from build123d import *

# Parameters (mm, degrees)
F0_R      = 31.75
F0_R_2    = 3.175
F1_DEPTH  = 12.7
F2_R      = 15.875
F2_R_2    = 9.525
F3_DEPTH  = 12.7
F3_FACE_R = 9.525
F4_DEPTH  = 25.4


with BuildPart() as f1:
    # F0 (on Top) → F1 (new body)
    with BuildSketch(Plane.XY):
        Circle(F0_R)
        with Locations((0, -25.4)):
            Circle(F0_R_2, mode=Mode.SUBTRACT)
        with Locations((-25.4, 0)):
            Circle(F0_R_2, mode=Mode.SUBTRACT)
        with Locations((25.4, 0)):
            Circle(F0_R_2, mode=Mode.SUBTRACT)
        with Locations((0, 25.4)):
            Circle(F0_R_2, mode=Mode.SUBTRACT)
    extrude(amount=F1_DEPTH)

    # F2 (on face) → F3 (join)
    with BuildSketch(Plane.XY.offset(12.7)):
        Circle(F2_R)
        Circle(F2_R_2, mode=Mode.SUBTRACT)
    extrude(amount=F3_DEPTH)

    # F3_face (on face) → F4 (cut)
    with BuildSketch(Plane.XY.offset(12.7)):
        Circle(F3_FACE_R)
    extrude(amount=-F4_DEPTH, mode=Mode.SUBTRACT)


solid = f1.part
Source: CAD feature listing. Evaluate the final solid. Frame: model axes, mm. A direction names the side the tool comes from. Round coordinates to 2 decimals unless told otherwise and drop trailing zeros. Write each loop counter-clockwise with the first axis right and the second up, starting at its lowest first coordinate (ties: lowest second). Pieces come first, ordered by that corner, then holes. Notation, with made-up numbers: (75.5, -0.5) - (82.5, -0.5) arc R20 ccw to (82.5, 19.5) - close; hole circle Ø3 at (8, 20). An arc over 180 degrees is marked (long way). Use CSV: the item, a comma, the result in double quotes. Start each with the question number.
(1) Material intervals for probe 1 along Y at (x, z) = (0, 9.75) (3 decimals); probe 2 along Y at (x, z) = (0, 22.75) (3 decimals); probe 3 along Z at (x, y) = (15, 22.5), sorted ascending. Write a range as [from, to].
(2) Cut plane D-D, the plane z = 8.75. Return loops of the section in (x, y) (3 decimals), and give its area (3 significant figures).
(3) Cut plane A-A, the plane x = 0. Return loops of the section in (y, z) (3 decimals).
(4) Mould query, pull axis X, two halves, no side actions, for faces 1 (the face through (7, 8, 0)), 2 (the face through (-0.41, -22.25, 6.26)), 3 (the face through (-3.441, -15.497, 18.961)). Classes: pulls with the +X half, pulls with the -X half, needs draft (parallel to the pull), parting line crosses it, or undercut.
(5) Set-up query: faces 4 (the face through (-6.883, -30.995, 6.261)), 5 (the face through (7, 15, 12.7)). Return all of +Z, -Z, +X, -X, +Y, -Y with unobstructed straight access to the full face (end or side cutting, diameter ignored); none if empty.
(6) Cut plane C-C, the plane x = -25.4. Return loops of the section in (y, z) (3 decimals).
(7) First-contact query: pin 1 Ø8.5 at (x, y) = (0, -25.4) entering from +Z; pin 2 Ø8 at (y, z) = (15.5, 6) entering from +X; pin 3 Ø12 at (y, z) = (15.5, 13) entering from -X. Flat tips, straight axial feed; report the tip coordinate or a pass-through.
Geometry says:
1,probe 1,"[-31.75, -28.575], [-22.225, -9.525], [9.525, 22.225], [28.575, 31.75]"
1,probe 2,"[-15.875, -9.525], [9.525, 15.875]"
1,probe 3,"[0, 12.7]"
2,outline,"circle Ø63.5 at (0, 0); hole circle Ø6.35 at (-25.4, 0); hole circle Ø19.05 at (0, 0); hole circle Ø6.35 at (0, -25.4); hole circle Ø6.35 at (0, 25.4); hole circle Ø6.35 at (25.4, 0)"
2,area,"2,760 mm²"
3,outline,"(-31.75, 0) - (-28.575, 0) - (-28.575, 12.7) - (-31.75, 12.7) - close; (-22.225, 0) - (-9.525, 0) - (-9.525, 25.4) - (-15.875, 25.4) - (-15.875, 12.7) - (-22.225, 12.7) - close; (9.525, 0) - (22.225, 0) - (22.225, 12.7) - (15.875, 12.7) - (15.875, 25.4) - (9.525, 25.4) - close; (28.575, 0) - (31.75, 0) - (31.75, 12.7) - (28.575, 12.7) - close"
4,face 1,"needs draft"
4,face 2,"undercut"
4,face 3,"parting line crosses it"
5,face 4,"+Z, -Z"
5,face 5,"+Z"
6,outline,"(-19.05, 0) - (-3.175, 0) - (-3.175, 12.7) - (-19.05, 12.7) - close; (3.175, 0) - (19.05, 0) - (19.05, 12.7) - (3.175, 12.7) - close"
7,pin 1,"z = 12.7"
7,pin 2,"x = 29.59"
7,pin 3,"x = -30.29"
